```python
from build123d import *

# Parameters (mm, degrees)
F1_DEPTH = 82.55
F2_R     = 3.81
F3_DEPTH = 25.4
F5_D     = 6.35
F5_DEPTH = 19.05
F5_TIP   = 1.9077324654


with BuildPart() as f1:
    # F0 (on Front) → F1 (new body)
    with BuildSketch(Plane.XZ):
        Polygon((0, 121.0280880332), (0, -12.3219119668), (38.1, -12.3219119668), (38.1, 141.0432880332), (20.0152, 141.0432880332), align=None)
    extrude(amount=F1_DEPTH)

    # F2 (on face) → F3 (cut)
    with BuildSketch(Plane(origin=(0, 0, -12.3219119668), x_dir=(1, 0, 0), z_dir=(0, 0, -1))):
        with Locations((19.05, 62.23)):
            Circle(F2_R)
        with Locations((19.05, 20.32)):
            Circle(F2_R)
    extrude(amount=-F3_DEPTH, mode=Mode.SUBTRACT)

    # F5
    with Locations(Plane(origin=(-60.5140440166, 0, 60.5140440166), x_dir=(0, -1, 0), z_dir=(-0.7071067812, 0, 0.7071067812))):
        with Locations((6.35, 99.7326654091), (69.85, 99.7326654091)):
            Hole(F5_D / 2, depth=F5_DEPTH)
            with Locations((0, 0, -(F5_DEPTH + F5_TIP / 2))):  # 118° drill point
                Cone(0, F5_D / 2, F5_TIP, mode=Mode.SUBTRACT)


solid = f1.part
```
Build history of the part. All positions in model axes, mm. A direction names the side the tool comes from. Give positions to 0.01 mm unless a question says otherwise; leave off trailing zeros. Loops run counter-clockwise (first coordinate to the right, second up) from the corner with the lowest first, then second, coordinate; pieces in that order, holes last.
1) Probe line 1 along Y through (x, z) = (19.05, -1.75); line 2 along X through (y, z) = (-20.32, -5); line 3 along Z through (x, y) = (22.5, -61.5). List the from-to ranges inside material, lowest first.
Values follow:
line 1: y = -82.55 to -66.04, -58.42 to -24.13, -16.51 to 0
line 2: x = 0 to 15.24, 22.86 to 38.1
line 3: z = 13.08 to 141.04
2) 3-axis set-ups, long thin cutter, end or side, ignore diameter. For faces 1 (the face through (0, -41, 55)), 2 (the face through (15.244, -20.488, 0.2)), 3 (the face through (24.247, -6.604, 116.105)): which of +Z, -Z, +X, -X, +Y, -Y reach the whole face in a straight line?
Values follow:
face 1: +Z, -Z, -X, +Y, -Y
face 2: -Z
face 3: none
3) Band-saw the part on B-B on y = -35.5. List the corners of the cut face in (x, z), then the cut area to 3 significant figures.
Values follow:
outline: (0, -12.32) - (38.1, -12.32) - (38.1, 141.04) - (20.02, 141.04) - (0, 121.03) - close
area: 5,640 mm2
4) Two-plate mould, pull along Z, no slides. Class faces 4 (the face through (18.22, -58.51, 0.2)), 5 (the face through (29, -41, 141.043)), 6 (the face through (24.4, -70.4, 116.3)): released by +Z, released by -Z, zero draft, split by the parting line, or undercut.
Values follow:
face 4: zero draft
face 5: released by +Z
face 6: undercut
5) Band-saw the part on A-A on y = -62.23. List the corners of the cut face in (x, z), then the cut area to 3 significant figures.
Values follow:
outline: (0, -12.32) - (15.24, -12.32) - (15.24, 13.08) - (22.86, 13.08) - (22.86, -12.32) - (38.1, -12.32) - (38.1, 141.04) - (20.02, 141.04) - (0, 121.03) - close
area: 5,450 mm2
6) Drop flat-ended pins along their axis: P1, Ø1, axis at x = 21.5, z = 7.5, coming from the +Y side; P2, Ø2.5, axis at x = 17.5, y = -63, coming from the -Z side; P3, Ø1.5, axis at x = 6.5, y = -42, coming from the +Z side; P4, Ø3, axis at x = 12, y = -72.5, coming from the +Z side. Give the stop position or say it passes through.
Values follow:
P1: stops at y = 0
P2: stops at z = 13.08
P3: stops at z = 128.28
P4: stops at z = 134.53
